from build123d import *

# Parameters (mm, degrees)
F0_R     = 2.2
F0_R_2   = 3.5
F1_DEPTH = 4
F2_DEPTH = 2.251


with BuildPart() as f1:
    # F0 (on Front) → F1 (new body)
    with BuildSketch(Plane.XZ):
        with BuildLine():
            Line((-38.1, 26.8488), (-38.1, 0))
            Line((-38.1, 0), (38.1, 0))
            Line((38.1, 0), (38.1, 26.8488))
            ThreePointArc((38.1, 26.8488), (37.147745567, 29.147745567), (34.8488, 30.1))
            Line((34.8488, 30.1), (-34.8488, 30.1))
            ThreePointArc((-34.8488, 30.1), (-37.147745567, 29.147745567), (-38.1, 26.8488))
        make_face()
        with BuildLine():
            Line((-34.8488, 26.8488), (-4.245966041, 26.8488))
            ThreePointArc((-4.245966041, 26.8488), (-0.75, 27.8), (2.745966041, 26.8488))
            Line((2.745966041, 26.8488), (24.754033959, 26.8488))
            ThreePointArc((24.754033959, 26.8488), (28.25, 27.8), (31.745966041, 26.8488))
            Line((31.745966041, 26.8488), (34.8488, 26.8488))
            Line((34.8488, 26.8488), (34.8488, 22.9163924618))
            ThreePointArc((34.8488, 22.9163924618), (35.0742845779, 21.9193821658), (35.15, 20.9))
            ThreePointArc((35.15, 20.9), (35.0742845779, 19.8806178342), (34.8488, 18.8836075382))
            Line((34.8488, 18.8836075382), (34.8488, 3.2512))
            Line((34.8488, 3.2512), (29.8756, 3.2512))
            Line((29.8756, 3.2512), (26.6244, 3.2512))
            Line((26.6244, 3.2512), (0.8756, 3.2512))
            Line((0.8756, 3.2512), (-2.3756, 3.2512))
            Line((-2.3756, 3.2512), (-34.8488, 3.2512))
            Line((-34.8488, 3.2512), (-34.8488, 26.8488))
        make_face(mode=Mode.SUBTRACT)
        with BuildLine():
            Line((-2.3756, 3.2512), (-2.3756, 14.194224531))
            ThreePointArc((-2.3756, 14.194224531), (-7.5758464496, 19.8911292219), (-4.245966041, 26.8488))
            Line((-4.245966041, 26.8488), (-34.8488, 26.8488))
            Line((-34.8488, 26.8488), (-34.8488, 3.2512))
            Line((-34.8488, 3.2512), (-2.3756, 3.2512))
        make_face()
        with Locations((-17.9, 10.074)):
            Circle(F0_R, mode=Mode.SUBTRACT)
        with Locations((-17.9, 21.074)):
            Circle(F0_R, mode=Mode.SUBTRACT)
        with BuildLine():
            ThreePointArc((6.15, 20.9), (4.6734048346, 16.6342433262), (0.8756, 14.194224531))
            Line((0.8756, 14.194224531), (0.8756, 3.2512))
            Line((0.8756, 3.2512), (26.6244, 3.2512))
            Line((26.6244, 3.2512), (26.6244, 14.194224531))
            ThreePointArc((26.6244, 14.194224531), (21.4241535504, 19.8911292219), (24.754033959, 26.8488))
            Line((24.754033959, 26.8488), (2.745966041, 26.8488))
            ThreePointArc((2.745966041, 26.8488), (5.2388298391, 24.3269399117), (6.15, 20.9))
        make_face()
        with BuildLine():
            ThreePointArc((-4.245966041, 26.8488), (-7.5758464496, 19.8911292219), (-2.3756, 14.194224531))
            ThreePointArc((-2.3756, 14.194224531), (-0.75, 14), (0.8756, 14.194224531))
            ThreePointArc((0.8756, 14.194224531), (4.6734048346, 16.6342433262), (6.15, 20.9))
            ThreePointArc((6.15, 20.9), (5.2388298391, 24.3269399117), (2.745966041, 26.8488))
            Line((2.745966041, 26.8488), (-4.245966041, 26.8488))
        make_face()
        with Locations((-0.75, 20.9)):
            Circle(F0_R_2, mode=Mode.SUBTRACT)
        with BuildLine():
            Line((31.745966041, 26.8488), (24.754033959, 26.8488))
            ThreePointArc((24.754033959, 26.8488), (21.4241535504, 19.8911292219), (26.6244, 14.194224531))
            ThreePointArc((26.6244, 14.194224531), (28.25, 14), (29.8756, 14.194224531))
            ThreePointArc((29.8756, 14.194224531), (32.9836843037, 15.8798174423), (34.8488, 18.8836075382))
            Line((34.8488, 18.8836075382), (34.8488, 22.9163924618))
            ThreePointArc((34.8488, 22.9163924618), (33.6668286494, 25.1741042784), (31.745966041, 26.8488))
        make_face()
        with Locations((28.25, 20.9)):
            Circle(F0_R_2, mode=Mode.SUBTRACT)
        with BuildLine():
            Line((29.8756, 14.194224531), (29.8756, 3.2512))
            Line((29.8756, 3.2512), (34.8488, 3.2512))
            Line((34.8488, 3.2512), (34.8488, 18.8836075382))
            ThreePointArc((34.8488, 18.8836075382), (32.9836843037, 15.8798174423), (29.8756, 14.194224531))
        make_face()
        with BuildLine():
            Line((26.6244, 14.194224531), (26.6244, 3.2512))
            Line((26.6244, 3.2512), (29.8756, 3.2512))
            Line((29.8756, 3.2512), (29.8756, 14.194224531))
            ThreePointArc((29.8756, 14.194224531), (28.25, 14), (26.6244, 14.194224531))
        make_face()
        with BuildLine():
            ThreePointArc((0.8756, 14.194224531), (-0.75, 14), (-2.3756, 14.194224531))
            Line((-2.3756, 14.194224531), (-2.3756, 3.2512))
            Line((-2.3756, 3.2512), (0.8756, 3.2512))
            Line((0.8756, 3.2512), (0.8756, 14.194224531))
        make_face()
        with BuildLine():
            Line((34.8488, 26.8488), (31.745966041, 26.8488))
            ThreePointArc((31.745966041, 26.8488), (33.6668286494, 25.1741042784), (34.8488, 22.9163924618))
            Line((34.8488, 22.9163924618), (34.8488, 26.8488))
        make_face()
        with BuildLine():
            ThreePointArc((31.745966041, 26.8488), (28.25, 27.8), (24.754033959, 26.8488))
            Line((24.754033959, 26.8488), (31.745966041, 26.8488))
        make_face()
        with BuildLine():
            ThreePointArc((2.745966041, 26.8488), (-0.75, 27.8), (-4.245966041, 26.8488))
            Line((-4.245966041, 26.8488), (2.745966041, 26.8488))
        make_face()
        with BuildLine():
            ThreePointArc((35.15, 20.9), (35.0742845779, 21.9193821658), (34.8488, 22.9163924618))
            Line((34.8488, 22.9163924618), (34.8488, 18.8836075382))
            ThreePointArc((34.8488, 18.8836075382), (35.0742845779, 19.8806178342), (35.15, 20.9))
        make_face()
    extrude(amount=F1_DEPTH)

    # F0 (on Front) → F2 (join)
    with BuildSketch(Plane.XZ):
        with BuildLine():
            Line((-38.1, 26.8488), (-38.1, 0))
            Line((-38.1, 0), (38.1, 0))
            Line((38.1, 0), (38.1, 26.8488))
            ThreePointArc((38.1, 26.8488), (37.147745567, 29.147745567), (34.8488, 30.1))
            Line((34.8488, 30.1), (-34.8488, 30.1))
            ThreePointArc((-34.8488, 30.1), (-37.147745567, 29.147745567), (-38.1, 26.8488))
        make_face()
        with BuildLine():
            Line((-34.8488, 26.8488), (-4.245966041, 26.8488))
            ThreePointArc((-4.245966041, 26.8488), (-0.75, 27.8), (2.745966041, 26.8488))
            Line((2.745966041, 26.8488), (24.754033959, 26.8488))
            ThreePointArc((24.754033959, 26.8488), (28.25, 27.8), (31.745966041, 26.8488))
            Line((31.745966041, 26.8488), (34.8488, 26.8488))
            Line((34.8488, 26.8488), (34.8488, 22.9163924618))
            ThreePointArc((34.8488, 22.9163924618), (35.0742845779, 21.9193821658), (35.15, 20.9))
            ThreePointArc((35.15, 20.9), (35.0742845779, 19.8806178342), (34.8488, 18.8836075382))
            Line((34.8488, 18.8836075382), (34.8488, 3.2512))
            Line((34.8488, 3.2512), (29.8756, 3.2512))
            Line((29.8756, 3.2512), (26.6244, 3.2512))
            Line((26.6244, 3.2512), (0.8756, 3.2512))
            Line((0.8756, 3.2512), (-2.3756, 3.2512))
            Line((-2.3756, 3.2512), (-34.8488, 3.2512))
            Line((-34.8488, 3.2512), (-34.8488, 26.8488))
        make_face(mode=Mode.SUBTRACT)
        with BuildLine():
            ThreePointArc((-4.245966041, 26.8488), (-7.5758464496, 19.8911292219), (-2.3756, 14.194224531))
            ThreePointArc((-2.3756, 14.194224531), (-0.75, 14), (0.8756, 14.194224531))
            ThreePointArc((0.8756, 14.194224531), (4.6734048346, 16.6342433262), (6.15, 20.9))
            ThreePointArc((6.15, 20.9), (5.2388298391, 24.3269399117), (2.745966041, 26.8488))
            Line((2.745966041, 26.8488), (-4.245966041, 26.8488))
        make_face()
        with Locations((-0.75, 20.9)):
            Circle(F0_R_2, mode=Mode.SUBTRACT)
        with BuildLine():
            ThreePointArc((0.8756, 14.194224531), (-0.75, 14), (-2.3756, 14.194224531))
            Line((-2.3756, 14.194224531), (-2.3756, 3.2512))
            Line((-2.3756, 3.2512), (0.8756, 3.2512))
            Line((0.8756, 3.2512), (0.8756, 14.194224531))
        make_face()
        with BuildLine():
            ThreePointArc((2.745966041, 26.8488), (-0.75, 27.8), (-4.245966041, 26.8488))
            Line((-4.245966041, 26.8488), (2.745966041, 26.8488))
        make_face()
        with BuildLine():
            Line((26.6244, 14.194224531), (26.6244, 3.2512))
            Line((26.6244, 3.2512), (29.8756, 3.2512))
            Line((29.8756, 3.2512), (29.8756, 14.194224531))
            ThreePointArc((29.8756, 14.194224531), (28.25, 14), (26.6244, 14.194224531))
        make_face()
        with BuildLine():
            Line((31.745966041, 26.8488), (24.754033959, 26.8488))
            ThreePointArc((24.754033959, 26.8488), (21.4241535504, 19.8911292219), (26.6244, 14.194224531))
            ThreePointArc((26.6244, 14.194224531), (28.25, 14), (29.8756, 14.194224531))
            ThreePointArc((29.8756, 14.194224531), (32.9836843037, 15.8798174423), (34.8488, 18.8836075382))
            Line((34.8488, 18.8836075382), (34.8488, 22.9163924618))
            ThreePointArc((34.8488, 22.9163924618), (33.6668286494, 25.1741042784), (31.745966041, 26.8488))
        make_face()
        with Locations((28.25, 20.9)):
            Circle(F0_R_2, mode=Mode.SUBTRACT)
        with BuildLine():
            ThreePointArc((31.745966041, 26.8488), (28.25, 27.8), (24.754033959, 26.8488))
            Line((24.754033959, 26.8488), (31.745966041, 26.8488))
        make_face()
        with BuildLine():
            Line((34.8488, 26.8488), (31.745966041, 26.8488))
            ThreePointArc((31.745966041, 26.8488), (33.6668286494, 25.1741042784), (34.8488, 22.9163924618))
            Line((34.8488, 22.9163924618), (34.8488, 26.8488))
        make_face()
        with BuildLine():
            ThreePointArc((35.15, 20.9), (35.0742845779, 21.9193821658), (34.8488, 22.9163924618))
            Line((34.8488, 22.9163924618), (34.8488, 18.8836075382))
            ThreePointArc((34.8488, 18.8836075382), (35.0742845779, 19.8806178342), (35.15, 20.9))
        make_face()
    extrude(amount=-F2_DEPTH)


solid = f1.part
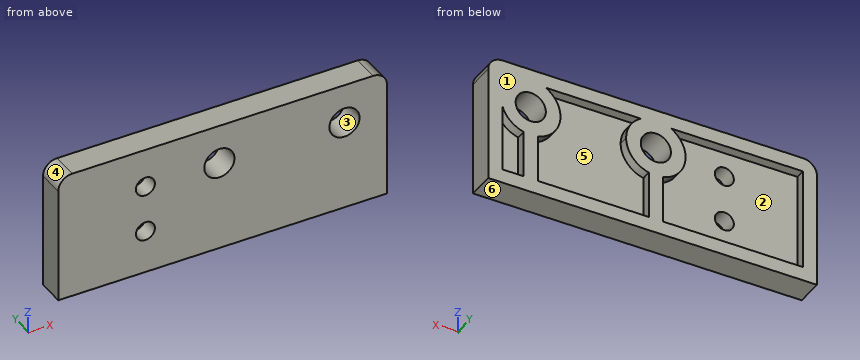
Build history of the part. All positions in model axes, mm. Face numbers are marked on the shaded views. A direction names the side the tool comes from. Give positions to 0.01 mm unless a question says otherwise; leave off trailing zeros. Write each loop counter-clockwise with the first axis right and the second up, starting at its lowest first coordinate (ties: lowest second). Pieces come first, ordered by that corner, then holes. Notation, with made-up numbers: (-27.75, 20.5) - (21.25, 20.5) arc R29 ccw to (21.25, 48.5) - close; hole circle Ø8 at (69, 49.5). An arc over 180 degrees is marked (long way). Use one line per item in the form item = value. Start each with the question number.
1. Probe line 1 (X direction, y = -3.5, z = 23.5); line 2 (Z direction, x = 1.5, y = 1.75); line 3 (X direction, y = -1.75, z = 22). List the from-to ranges inside material, lowest first. Write a range as [from, to].
2. Band-saw the part on D-D on x = 17. Write the cut outline in (y, z), plus the area to 3 significant figures.
3. 3-axis set-ups, long thin cutter, end or side, ignore diameter. For the marked faces 1 and 2: which of +Z, -Z, +X, -X, +Y, -Y reach the whole face in a straight line?
4. Band-saw the part on A-A on x = -0.75. Write the cut outline in (y, z).
5. Band-saw the part on B-B on y = 1. Write the cut outline in (x, z), plus the area to 3 significant figures.
6. Two-plate mould, pull along X, no slides. Class the marked faces 3, 4, 5 and 6: released by +X, released by -X, zero draft, split by the parting line, or undercut.
7. Drop a flat-ended pin along its axis: pin 1 Ø4 at (x, z) = (20, 13.5) entering from +Y. Give the stop position or say it passes through.
8. Band-saw the part on C-C on x = -17.9. Write the cut outline in (y, z).
Conclusion:
q1.line_1 = [-38.1, -3.09], [1.59, 25.91], [30.59, 38.1]
q1.line_2 = [0, 3.25], [14.38, 18.22], [23.58, 30.1]
q1.line_3 = [-38.1, -19.9], [-15.9, -4.07], [2.57, 24.93], [31.57, 38.1]
q2.outline = (-4, 0) - (2.25, 0) - (2.25, 3.25) - (0, 3.25) - (0, 26.85) - (2.25, 26.85) - (2.25, 30.1) - (-4, 30.1) - close
q2.area = 135 mm²
q3.face_1 = +Z, -Z, +X, -X, +Y
q3.face_2 = +Y
q4.outline = (-4, 0) - (2.25, 0) - (2.25, 17.4) - (-4, 17.4) - close; (-4, 24.4) - (2.25, 24.4) - (2.25, 30.1) - (-4, 30.1) - close
q5.outline = (-38.1, 0) - (38.1, 0) - (38.1, 26.85) arc R3.25 ccw to (34.85, 30.1) - (-34.85, 30.1) arc R3.25 ccw to (-38.1, 26.85) - close; hole (-34.85, 3.25) - (-2.38, 3.25) - (-2.38, 14.19) arc R6.9 cw to (-4.25, 26.85) - (-34.85, 26.85) - close; hole circle Ø7 at (-0.75, 20.9); hole (0.88, 3.25) - (26.62, 3.25) - (26.62, 14.19) arc R6.9 cw to (24.75, 26.85) - (2.75, 26.85) arc R6.9 cw to (0.88, 14.19) - close; hole circle Ø7 at (28.25, 20.9); hole (29.88, 3.25) - (34.85, 3.25) - (34.85, 18.88) arc R6.9 cw to (29.88, 14.19) - close
q5.area = 932 mm²
q6.face_3 = undercut
q6.face_4 = released by -X
q6.face_5 = undercut
q6.face_6 = zero draft
q7.pin_1 = 0
q8.outline = (-4, 0) - (2.25, 0) - (2.25, 3.25) - (0, 3.25) - (0, 7.87) - (-4, 7.87) - close; (-4, 12.27) - (0, 12.27) - (0, 18.87) - (-4, 18.87) - close; (-4, 23.27) - (0, 23.27) - (0, 26.85) - (2.25, 26.85) - (2.25, 30.1) - (-4, 30.1) - close
